Autodesk Inventor part; units mm, degrees
ref_plane "YZ Plane" through (0, 0, 0) normal (1, 0, 0) x (0, 1, 0)
ref_plane "XZ Plane" through (0, 0, 0) normal (0, 1, 0) x (-1, 0, 0)
ref_plane "XY Plane" through (0, 0, 0) normal (0, 0, 1) x (1, 0, 0)
sketch "Sketch1" plane through (0, 0, 0) normal (0, 1, 0) x (-1, 0, 0)
  line L0 (17.4506, 75.8516) -> (-84.1494, 75.8516)
  line L1 (-84.1494, 75.8516) -> (-84.1494, -25.7484)
  line L2 (-84.1494, -25.7484) -> (17.4506, -25.7484)
  line L3 (17.4506, -25.7484) -> (17.4506, 75.8516)
  point P0 (0, 0)
  dimension "d0" = 101.6
  dimension "d1" = 101.6
extrude "Extrusion1" add sketch "Sketch1" along normal blind 203.2
sketch "Sketch2" plane through (-17.4506, 0, 75.8516) normal (0, 0, 1) x (1, 0, 0)
  line L0 (0, 0) -> (0, 203.2)
  line L1 (101.6, 0) -> (101.6, 203.2)
  line L2 (0, 190.6053) -> (101.6, 190.6053)
  line L3 (101.6, 190.6053) -> (101.6, 155.0988)
  line L4 (101.6, 155.0988) -> (0, 155.0988)
  line L5 (0, 155.0988) -> (0, 190.6053)
  point P0 (17.4506, 0)
  point P1 (0, 155.0988)
  point P2 (101.6, 190.6053)
extrude "Extrusion2" cut sketch "Sketch2" against normal blind 96.52
sketch "Sketch3" plane through (-17.4506, 203.2, 75.8516) normal (0, 0, 1) x (1, 0, 0)
  circle A0 centre (6.9601, -5.4934) radius 5.1747
  circle A1 centre (31.169, -5.4934) radius 4.519
  circle A2 centre (56.0236, -5.4934) radius 4.519
  circle A3 centre (85.0743, -5.4934) radius 4.1962
  point P0 (17.4506, -203.2)
extrude "Extrusion3" cut sketch "Sketch3" against normal blind 8.89
sketch "Sketch4" plane through (-17.4506, 0, 75.8516) normal (0, 0, 1) x (1, 0, 0)
  line L0 (8.574, 144.124) -> (37.6248, 144.124)
  line L1 (37.6248, 144.124) -> (37.6248, 118.3011)
  line L2 (37.6248, 118.3011) -> (8.574, 118.3011)
  line L3 (8.574, 118.3011) -> (8.574, 144.124)
  line L4 (57.3147, 144.124) -> (89.2705, 144.124)
  line L5 (89.2705, 144.124) -> (89.2705, 118.3011)
  line L6 (89.2705, 118.3011) -> (57.3147, 118.3011)
  line L7 (57.3147, 118.3011) -> (57.3147, 144.124)
  line L8 (8.574, 91.1871) -> (37.6248, 91.1871)
  line L9 (37.6248, 91.1871) -> (37.6248, 65.0414)
  line L10 (37.6248, 65.0414) -> (8.574, 65.0414)
  line L11 (8.574, 65.0414) -> (8.574, 91.1871)
  line L12 (57.3147, 91.1871) -> (89.2705, 91.1871)
  line L13 (89.2705, 91.1871) -> (89.2705, 61.4908)
  line L14 (89.2705, 61.4908) -> (57.3147, 61.4908)
  line L15 (57.3147, 61.4908) -> (57.3147, 91.1871)
  point P0 (17.4506, 0)
extrude "Extrusion4" cut sketch "Sketch4" against normal blind 38.1
sketch "Sketch5" plane through (-17.4506, 0, 75.8516) normal (0, 0, 1) x (1, 0, 0)
  line L0 (87.4727, 45.3482) -> (87.4727, 27.2761)
  line L1 (87.4727, 27.2761) -> (91.8686, 27.2761)
  line L2 (91.8686, 27.2761) -> (91.8686, 45.3482)
  line L3 (91.8686, 45.3482) -> (87.4727, 45.3482)
  point P0 (17.4506, 0)
extrude "Extrusion5" cut sketch "Sketch5" against normal blind 25.4
sketch "Sketch6" plane through (-17.4506, 0, 75.8516) normal (0, 0, 1) x (1, 0, 0)
  line L0 (3.0866, 15.6551) -> (97.663, 15.6551)
  line L1 (97.663, 15.6551) -> (97.663, 2.0981)
  line L2 (97.663, 2.0981) -> (3.0866, 2.0981)
  line L3 (3.0866, 2.0981) -> (3.0866, 15.6551)
  point P0 (17.4506, 0)
extrude "Extrusion6" add sketch "Sketch6" along normal blind 30.48
sketch "Sketch7" plane through (-17.4506, 0, 75.8516) normal (0, 0, 1) x (1, 0, 0)
  line L0 (10.1224, 40.7313) -> (31.5958, 40.7313)
  line L1 (31.5958, 40.7313) -> (31.5958, 25.3932)
  line L2 (31.5958, 25.3932) -> (10.1224, 25.3932)
  line L3 (10.1224, 25.3932) -> (10.1224, 40.7313)
  point P0 (17.4506, 0)
extrude "Extrusion7" add sketch "Sketch7" along normal blind 22.86
sketch "Sketch8" plane through (-17.4506, 0, 37.7516) normal (0, 0, 1) x (1, 0, 0)
  line L0 (18.3983, 134.6076) -> (29.055, 134.6076)
  line L1 (29.055, 134.6076) -> (29.055, 130.1851)
  line L2 (29.055, 130.1851) -> (18.3983, 130.1851)
  line L3 (18.3983, 130.1851) -> (18.3983, 134.6076)
  point P0 (17.4506, 0)
extrude "Extrusion8" add sketch "Sketch8" along normal blind 22.86
sketch "Sketch9" plane through (-17.4506, 0, 37.7516) normal (0, 0, 1) x (1, 0, 0)
  line L0 (68.4801, 134.1332) -> (78.7235, 134.1332)
  line L1 (78.7235, 134.1332) -> (78.7235, 130.0548)
  line L2 (78.7235, 130.0548) -> (68.4801, 130.0548)
  line L3 (68.4801, 130.0548) -> (68.4801, 134.1332)
  point P0 (17.4506, 0)
extrude "Extrusion9" add sketch "Sketch9" along normal blind 22.86
sketch "Sketch10" plane through (-17.4506, 0, 37.7516) normal (0, 0, 1) x (1, 0, 0)
  line L0 (16.1934, 82.4203) -> (27.2154, 82.4203)
  line L1 (27.2154, 82.4203) -> (27.2154, 79.0146)
  line L2 (27.2154, 79.0146) -> (16.1934, 79.0146)
  line L3 (16.1934, 79.0146) -> (16.1934, 82.4203)
  point P0 (17.4506, 0)
extrude "Extrusion10" add sketch "Sketch10" along normal blind 22.86
sketch "Sketch11" plane through (-17.4506, 0, 37.7516) normal (0, 0, 1) x (1, 0, 0)
  line L0 (67.5137, 81.9751) -> (79.9385, 81.9751)
  line L1 (79.9385, 81.9751) -> (79.9385, 78.1143)
  line L2 (79.9385, 78.1143) -> (67.5137, 78.1143)
  line L3 (67.5137, 78.1143) -> (67.5137, 81.9751)
  point P0 (17.4506, 0)
extrude "Extrusion11" add sketch "Sketch11" along normal blind 22.86
sketch "Sketch12" plane through (-17.4506, 0, 60.6116) normal (0, 0, 1) x (1, 0, 0)
  line L0 (15.1277, 133.0839) -> (32.1051, 133.0839)
  line L1 (32.1051, 133.0839) -> (32.1051, 131.5664)
  line L2 (32.1051, 131.5664) -> (15.1277, 131.5664)
  line L3 (15.1277, 131.5664) -> (15.1277, 133.0839)
  point P0 (17.4506, 0)
extrude "Extrusion12" add sketch "Sketch12" along normal blind 25.4
sketch "Sketch13" plane through (-17.4506, 0, 60.6116) normal (0, 0, 1) x (1, 0, 0)
  line L0 (66.7886, 132.615) -> (80.7539, 132.615)
  line L1 (80.7539, 132.615) -> (80.7539, 131.3454)
  line L2 (80.7539, 131.3454) -> (66.7886, 131.3454)
  line L3 (66.7886, 131.3454) -> (66.7886, 132.615)
  point P0 (17.4506, 0)
extrude "Extrusion13" add sketch "Sketch13" along normal blind 25.4
sketch "Sketch14" plane through (-17.4506, 0, 60.6116) normal (0, 0, 1) x (1, 0, 0)
  line L0 (14.3022, 80.9529) -> (29.0306, 80.9529)
  line L1 (29.0306, 80.9529) -> (29.0306, 79.8856)
  line L2 (29.0306, 79.8856) -> (14.3022, 79.8856)
  line L3 (14.3022, 79.8856) -> (14.3022, 80.9529)
  point P0 (17.4506, 0)
extrude "Extrusion14" add sketch "Sketch14" along normal blind 25.4
sketch "Sketch15" plane through (-17.4506, 0, 60.6116) normal (0, 0, 1) x (1, 0, 0)
  line L0 (66.065, 80.6327) -> (82.2876, 80.6327)
  line L1 (82.2876, 80.6327) -> (82.2876, 79.1385)
  line L2 (82.2876, 79.1385) -> (66.065, 79.1385)
  line L3 (66.065, 79.1385) -> (66.065, 80.6327)
  point P0 (17.4506, 0)
extrude "Extrusion15" add sketch "Sketch15" along normal blind 25.4
sketch "Sketch16" plane through (-17.4506, 155.0988, 75.8516) normal (0, 1, 0) x (1, 0, 0)
  point P0 (17.4506, 75.8516)
properties part number "fff"
Build history of the part. All positions in model axes, mm. A direction names the side the tool comes from. Round coordinates to 2 decimals unless told otherwise and drop trailing zeros. Order: outer loops, then holes, each group sorted by start corner. A loop starts at its lowest first (then second) coordinate and runs counter-clockwise, first axis right, second up. Notation, with made-up numbers: M 82,87.5 L 134,87.5 A28 ccw 134,121.5 Z; hole C -37,5 d4. An arc over 180 degrees is marked long. Use CSV: the item, a comma, the result in double quotes. Start each with the question number.
(1) Flat gauge pins, fed straight in: P1, Ø1.2, axis at y = 132.5, z = 77.5, coming from the -X side; P2, Ø13, axis at x = 55.5, y = 137.5, coming from the +Z side; P3, Ø15, axis at y = 11, z = 90, coming from the -X side; P4, Ø5, axis at x = 38, z = 40, coming from the -Y side. Where does each tip first touch, or does it go through?
(2) Cut at D-D on y = 21.5. List the corners of the cut face in (x, z).
(3) Cut at B-B on x = 28.5. List the corners of the cut face in (y, z), then the cut area to 3 significant figures.
(4) Cut at A-A on z = 92.5. List the corners of the cut face in (x, y), then the cut area to 3 significant figures.
(5) Cut at C-C on z = 18. List the corners of the cut face in (x, y).
(6) Drill centre lines: probe 1 along X at (y, z) = (128, 57.5); probe 2 along Y at (x, z) = (62, 49.5); probe 3 along Y at (x, z) = (53, 67.5) (1 decimal). Where is each one in solid material? Low to high.
(7) Mould opens along Y. For faces 5 (the face through (-17.451, 78, 24)), 6 (the face through (56, 131.345, 73)), 7 (the face through (34, 203.2, 26)) say: +Y half, -Y half, draft (parallel to the pull), parting line (faces both ways), or undercut.
(8) Tool access for faces 1 (the face through (34, 100, -25.748)), 2 (the face through (3, 40.731, 87)), 3 (the face through (-11.612, 192.655, 71.469)), 4 (the face through (33, 197, 75.852)): list every direction of +Z, -Z, +X, -X, +Y, -Y with a clear straight run to the whole face (end or side of a thin tool).
Findings:
1,P1,"stops at x = -2.32"
1,P2,"stops at z = 86.01"
1,P3,"stops at x = -14.36"
1,P4,"stops at y = 0"
2,outline,"M -17.45,-25.75 L 84.15,-25.75 L 84.15,75.85 L -17.45,75.85 Z"
3,outline,"M 0,-25.75 L 203.2,-25.75 L 203.2,75.85 L 190.61,75.85 L 190.61,-20.67 L 155.1,-20.67 L 155.1,75.85 L 15.66,75.85 L 15.66,106.33 L 2.1,106.33 L 2.1,75.85 L 0,75.85 Z"
3,area,"17,600 mm^2"
4,outline,"M -14.36,2.1 L 80.21,2.1 L 80.21,15.66 L -14.36,15.66 Z; M -7.33,25.39 L 14.15,25.39 L 14.15,40.73 L -7.33,40.73 Z"
4,area,"1,610 mm^2"
5,outline,"M -17.45,0 L 84.15,0 L 84.15,155.1 L -17.45,155.1 Z; M -17.45,190.61 L 84.15,190.61 L 84.15,203.2 L -17.45,203.2 Z"
6,probe 1,"x = -17.45 to -8.88, 20.17 to 39.86, 71.82 to 84.15"
6,probe 2,"y = 0 to 61.49, 78.11 to 81.98, 91.19 to 118.3, 144.12 to 155.1, 190.61 to 203.2"
6,probe 3,"y = 0 to 61.5, 79.1 to 80.6, 91.2 to 118.3, 131.3 to 132.6, 144.1 to 155.1, 190.6 to 203.2"
7,face 5,"draft"
7,face 6,"undercut"
7,face 7,"+Y half"
8,face 1,"-Z, +X, -X, +Y, -Y"
8,face 2,"+Z, +X, -X"
8,face 3,"+Z"
8,face 4,"+Z, +X, -X, +Y"
